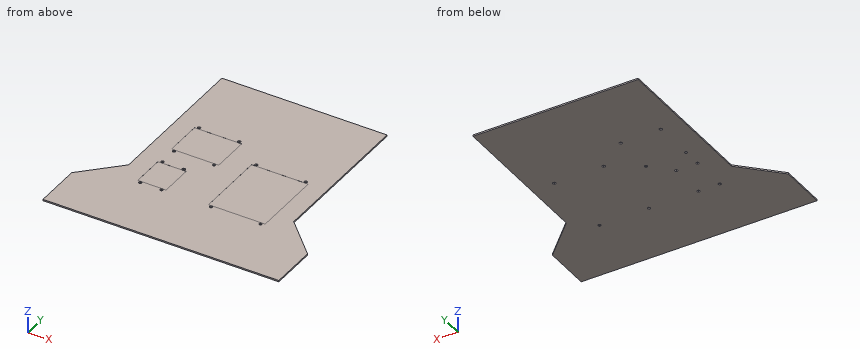
from build123d import *

# Parameters (mm, degrees)
BOSS_EXTRUDE1_DEPTH = 3
CUT_EXTRUDE3_START  = 3
SKETCH3_W           = 100
SKETCH3_H           = 80
SKETCH3_W_2         = 120
SKETCH3_H_2         = 150
SKETCH3_W_3         = 60
SKETCH3_H_3         = 70
CUT_EXTRUDE3_DEPTH  = 0.1
CUT_EXTRUDE4_DEPTH  = 560.025044162


with BuildPart() as part:
    # Sketch1 → Boss-Extrude1 (new body)
    with BuildSketch(Plane.XY):
        Polygon((-250, 0), (-250, 100), (-175, 175), (-175, 500), (175, 500), (175, 175), (250, 100), (250, 0), align=None)
    extrude(amount=BOSS_EXTRUDE1_DEPTH)

    # Sketch3 → Cut-Extrude3 (cut)
    with BuildSketch(Plane.XY.offset(CUT_EXTRUDE3_START)):
        with Locations((-85, 298.75)):
            Rectangle(SKETCH3_W, SKETCH3_H)
        with Locations((75, 216.25)):
            Rectangle(SKETCH3_W_2, SKETCH3_H_2)
        with Locations((-105, 176.25)):
            Rectangle(SKETCH3_W_3, SKETCH3_H_3)
    extrude(amount=-CUT_EXTRUDE3_DEPTH, mode=Mode.SUBTRACT)

    # Sketch4 → Cut-Extrude4 (cut, through all)
    with BuildSketch(Plane(origin=(0, 0, 0), x_dir=(-1, 0, 0), z_dir=(0, 0, -1))):
        Polygon((-20.767949192, 140.5), (-24.232050808, 140.5), (-25.964101615, 137.5), (-24.232050808, 134.5), (-20.767949192, 134.5), (-19.035898385, 137.5), align=None)
        Polygon((-129.232050808, 134.5), (-125.767949192, 134.5), (-124.035898385, 137.5), (-125.767949192, 140.5), (-129.232050808, 140.5), (-130.964101615, 137.5), align=None)
        Polygon((79.035898385, 137.5), (80.767949192, 134.5), (84.232050808, 134.5), (85.964101615, 137.5), (84.232050808, 140.5), (80.767949192, 140.5), align=None)
        Polygon((129.232050808, 134.5), (130.964101615, 137.5), (129.232050808, 140.5), (125.767949192, 140.5), (124.035898385, 137.5), (125.767949192, 134.5), align=None)
        Polygon((129.232050808, 218), (125.767949192, 218), (124.035898385, 215), (125.767949192, 212), (129.232050808, 212), (130.964101615, 215), align=None)
        Polygon((80.767949192, 218), (79.035898385, 215), (80.767949192, 212), (84.232050808, 212), (85.964101615, 215), (84.232050808, 218), align=None)
        Polygon((125.767949192, 252), (129.232050808, 252), (130.964101615, 255), (129.232050808, 258), (125.767949192, 258), (124.035898385, 255), align=None)
        Polygon((44.232050808, 252), (45.964101615, 255), (44.232050808, 258), (40.767949192, 258), (39.035898385, 255), (40.767949192, 252), align=None)
        Polygon((-130.964101615, 295), (-129.232050808, 292), (-125.767949192, 292), (-124.035898385, 295), (-125.767949192, 298), (-129.232050808, 298), align=None)
        Polygon((-19.035898385, 295), (-20.767949192, 298), (-24.232050808, 298), (-25.964101615, 295), (-24.232050808, 292), (-20.767949192, 292), align=None)
        Polygon((40.767949192, 345.5), (39.035898385, 342.5), (40.767949192, 339.5), (44.232050808, 339.5), (45.964101615, 342.5), (44.232050808, 345.5), align=None)
        Polygon((129.232050808, 345.5), (125.767949192, 345.5), (124.035898385, 342.5), (125.767949192, 339.5), (129.232050808, 339.5), (130.964101615, 342.5), align=None)
    extrude(amount=-CUT_EXTRUDE4_DEPTH, mode=Mode.SUBTRACT)


solid = part.part
The model under review builds one solid part; all positions refer to its coordinate system, in mm. Round coordinates to 2 decimals unless told otherwise and drop trailing zeros. Loops run counter-clockwise (first coordinate to the right, second up) from the corner with the lowest first, then second, coordinate; pieces in that order, holes last. Notation, with made-up numbers: (-1, 85) -> (44, 85) arc R21 cw to (44, 116) -> close; hole circle Ø5 at (38, 3.5). An arc over 180 degrees is marked (long way). Answer as CSV lines item,"result".
1) Add section A-A on y = 187. Write out the cut boundary in (x, z).
Geometry results:
outline,"(-175, 0) -> (175, 0) -> (175, 3) -> (135, 3) -> (135, 2.9) -> (15, 2.9) -> (15, 3) -> (-75, 3) -> (-75, 2.9) -> (-135, 2.9) -> (-135, 3) -> (-175, 3) -> close"
2) Add section D-D on y = 307. Write out the cut boundary in (x, z).
Geometry results:
outline,"(-175, 0) -> (175, 0) -> (175, 3) -> (-35, 3) -> (-35, 2.9) -> (-135, 2.9) -> (-135, 3) -> (-175, 3) -> close"
3) Add section B-B on z = 0.8. State how many separate pieces and enclosed holes the cut face has, plus the area to 3 significant figures.
Geometry results:
separate pieces,"1"
enclosed holes,"12"
area,"195,000 mm²"
4) Add section C-C on x = 202. Write out the cut boundary in (y, z).
Geometry results:
outline,"(0, 0) -> (148, 0) -> (148, 3) -> (0, 3) -> close"
5) For P1, Ø1.5, axis at y = 342, z = 2, coming from the +X side; P2, Ø1, axis at y = 446.5, z = 1.5, coming from the -X side; P3, Ø1.5, axis at y = 108.5, z = 2.5, coming from the -X side, all flat-tipped, find the tip position at first contact; note any pin that passes through.
Geometry results:
P1,"stops at x = 175"
P2,"stops at x = -175"
P3,"stops at x = -242.25"
6) To check wall thickness, follow line 1 along Y through (x, z) = (-128, 1.9); line 2 along Y through (x, z) = (128, 0.3); line 3 along X through (y, z) = (216, 2.45). State the ranges of each line that lie inside material, in increasing order. Write a range as from..to.
Geometry results:
line 1,"y = 0..134.5, 140.5..212, 218..252, 258..339.5, 345.5..500"
line 2,"y = 0..134.5, 140.5..292, 298..500"
line 3,"x = -175..-130.39, -124.61..-85.39, -79.61..175"
